Source: CAD feature listing. Evaluate the final solid. Frame: model axes, mm. Coordinates: 2 decimals unless noted, no trailing zeros. Loops run counter-clockwise (first coordinate to the right, second up) from the corner with the lowest first, then second, coordinate; pieces in that order, holes last. Notation, with made-up numbers: (65, -34.5) -> (83, -34.5) arc R19 ccw to (83, -24.5) -> close; hole circle Ø11 at (80.25, -35.75). An arc over 180 degrees is marked (long way). Answer as CSV lines item,"result".
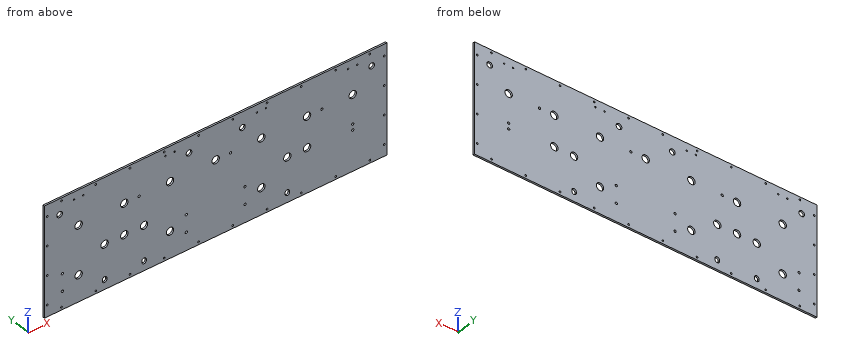
from build123d import *

# Parameters (mm, degrees)
SKETCH1_W           = 600
SKETCH1_H           = 190
EXTRUDE1_DEPTH      = 3
SKETCH2_R           = 6.5
CUT_EXTRUDE1_DEPTH  = 614.929149007
SKETCH5_R           = 2
CUT_EXTRUDE3_DEPTH  = 614.929149007
SKETCH8_R           = 6.5
SKETCH8_R_2         = 2
CUT_EXTRUDE4_DEPTH  = 614.929149007
SKETCH10_R          = 6.5
CUT_EXTRUDE5_DEPTH  = 614.929149007
SKETCH12_R          = 6.5
CUT_EXTRUDE6_DEPTH  = 614.929149007
SKETCH14_R          = 1.25
CUT_EXTRUDE7_DEPTH  = 614.929149007
SKETCH15_R          = 5
CUT_EXTRUDE8_DEPTH  = 614.929149007
CUT_EXTRUDE10_DEPTH = 614.929149007
SKETCH25_R          = 1.5
CUT_EXTRUDE11_DEPTH = 614.929149007
LPATTERN1_COUNT     = 10
LPATTERN1_PITCH     = 60
SKETCH26_R          = 1.5
CUT_EXTRUDE12_DEPTH = 614.929149007
SKETCH27_R          = 2
CUT_EXTRUDE13_DEPTH = 614.929149007


with BuildPart() as part:
    # Sketch1 → Extrude1 (new body)
    with BuildSketch(Plane(origin=(0, 0, 0), x_dir=(1, 0, 0), z_dir=(0, 1, 0))):
        with Locations((300, 35)):
            Rectangle(SKETCH1_W, SKETCH1_H)
    extrude(amount=EXTRUDE1_DEPTH)

    # Sketch2 → Cut-Extrude1 (cut, through all)
    with BuildSketch(Plane(origin=(0, 3, 0), x_dir=(-1, 0, 0), z_dir=(0, 1, 0))):
        with Locations(Location((-60, 0, 0), (0, 0, 90))):
            Circle(SKETCH2_R)
        with Locations(Location((-140, 0, 0), (0, 0, 90))):
            Circle(SKETCH2_R)
        with Locations(Location((-220, 0, 0), (0, 0, 90))):
            Circle(SKETCH2_R)
        with Locations(Location((-300, 0, 0), (0, 0, 90))):
            Circle(SKETCH2_R)
        with Locations(Location((-380, 0, 0), (0, 0, 90))):
            Circle(SKETCH2_R)
        with Locations(Location((-460, 0, 0), (0, 0, 90))):
            Circle(SKETCH2_R)
        with Locations(Location((-540, 0, 0), (0, 0, 90))):
            Circle(SKETCH2_R)
    extrude(amount=-CUT_EXTRUDE1_DEPTH, mode=Mode.SUBTRACT)

    # Sketch5 → Cut-Extrude3 (cut, through all)
    with BuildSketch(Plane(origin=(0, 3, 0), x_dir=(-1, 0, 0), z_dir=(0, 1, 0))):
        with Locations(Location((-166, 0, 0), (0, 0, 90))):
            Circle(SKETCH5_R)
        with Locations(Location((-326, 0, 0), (0, 0, 90))):
            Circle(SKETCH5_R)
        with Locations(Location((-486, 0, 0), (0, 0, 90))):
            Circle(SKETCH5_R)
    extrude(amount=-CUT_EXTRUDE3_DEPTH, mode=Mode.SUBTRACT)

    # Sketch8 → Cut-Extrude4 (cut, through all)
    with BuildSketch(Plane(origin=(0, 3, 0), x_dir=(-1, 0, 0), z_dir=(0, 1, 0))):
        with Locations(Location((-105.461363383, -53.228417592, 0), (0, 0, 90))):
            Circle(SKETCH8_R)
        with Locations(Location((-540, -60, 0), (0, 0, 90))):
            Circle(SKETCH8_R_2)
        with Locations(Location((-425.461363383, -53.228417592, 0), (0, 0, 90))):
            Circle(SKETCH8_R)
        with Locations(Location((-174.538636617, -53.228417592, 0), (0, 0, 90))):
            Circle(SKETCH8_R)
        with Locations(Location((-540, -50, 0), (0, 0, 90))):
            Circle(SKETCH8_R_2)
    extrude(amount=-CUT_EXTRUDE4_DEPTH, mode=Mode.SUBTRACT)

    # Sketch10 → Cut-Extrude5 (cut, through all)
    with BuildSketch(Plane(origin=(0, 3, 0), x_dir=(-1, 0, 0), z_dir=(0, 1, 0))):
        with Locations(Location((-60, -84.184264202, 0), (0, 0, 90))):
            Circle(SKETCH10_R)
        with Locations(Location((-220, -84.184264202, 0), (0, 0, 90))):
            Circle(SKETCH10_R)
        with Locations(Location((-380, -84.184264202, 0), (0, 0, 90))):
            Circle(SKETCH10_R)
    extrude(amount=-CUT_EXTRUDE5_DEPTH, mode=Mode.SUBTRACT)

    # Sketch12 → Cut-Extrude6 (cut, through all)
    with BuildSketch(Plane(origin=(0, 3, 0), x_dir=(-1, 0, 0), z_dir=(0, 1, 0))):
        with Locations(Location((-140, -53.228417592, 0), (0, 0, 90))):
            Circle(SKETCH12_R)
        with Locations(Location((-460, -53.228417592, 0), (0, 0, 90))):
            Circle(SKETCH12_R)
    extrude(amount=-CUT_EXTRUDE6_DEPTH, mode=Mode.SUBTRACT)

    # Sketch14 → Cut-Extrude7 (cut, through all)
    with BuildSketch(Plane(origin=(0, 3, 0), x_dir=(-1, 0, 0), z_dir=(0, 1, 0))):
        with Locations(Location((-52, 47, 0), (0, 0, 90))):
            Circle(SKETCH14_R)
        with Locations(Location((-68, 47, 0), (0, 0, 90))):
            Circle(SKETCH14_R)
        with Locations(Location((-212, 47, 0), (0, 0, 90))):
            Circle(SKETCH14_R)
        with Locations(Location((-228, 47, 0), (0, 0, 90))):
            Circle(SKETCH14_R)
        with Locations(Location((-372, 47, 0), (0, 0, 90))):
            Circle(SKETCH14_R)
        with Locations(Location((-388, 47, 0), (0, 0, 90))):
            Circle(SKETCH14_R)
        with Locations(Location((-532, 47, 0), (0, 0, 90))):
            Circle(SKETCH14_R)
        with Locations(Location((-548, 47, 0), (0, 0, 90))):
            Circle(SKETCH14_R)
    extrude(amount=-CUT_EXTRUDE7_DEPTH, mode=Mode.SUBTRACT)

    # Sketch15 → Cut-Extrude8 (cut, through all)
    with BuildSketch(Plane(origin=(0, 3, 0), x_dir=(-1, 0, 0), z_dir=(0, 1, 0))):
        with Locations(Location((-573.234018716, 33.234018716, 0), (0, 0, 90))):
            Circle(SKETCH15_R)
        with Locations(Location((-26.765981284, 33.234018716, 0), (0, 0, 90))):
            Circle(SKETCH15_R)
        with Locations(Location((-253.234018716, 33.234018716, 0), (0, 0, 90))):
            Circle(SKETCH15_R)
        with Locations(Location((-346.765981284, 33.234018716, 0), (0, 0, 90))):
            Circle(SKETCH15_R)
    extrude(amount=-CUT_EXTRUDE8_DEPTH, mode=Mode.SUBTRACT)

    # Sketch23 → Cut-Extrude10 (cut, through all)
    with BuildSketch(Plane(origin=(0, 3, 0), x_dir=(-1, 0, 0), z_dir=(0, 1, 0))):
        with BuildLine():
            Line((-101.461363383, -112.228417592), (-101.461363383, -114.228417592))
            ThreePointArc((-101.461363383, -114.228417592), (-105.461363383, -118.228417592), (-109.461363383, -114.228417592))
            Line((-109.461363383, -114.228417592), (-109.461363383, -112.228417592))
            ThreePointArc((-109.461363383, -112.228417592), (-105.461363383, -108.228417592), (-101.461363383, -112.228417592))
        make_face()
        with BuildLine():
            Line((-170.538636617, -112.228417592), (-170.538636617, -114.228417592))
            ThreePointArc((-170.538636617, -114.228417592), (-174.538636617, -118.228417592), (-178.538636617, -114.228417592))
            Line((-178.538636617, -114.228417592), (-178.538636617, -112.228417592))
            ThreePointArc((-178.538636617, -112.228417592), (-174.538636617, -108.228417592), (-170.538636617, -112.228417592))
        make_face()
        with BuildLine():
            Line((-421.461363383, -112.228417592), (-421.461363383, -114.228417592))
            ThreePointArc((-421.461363383, -114.228417592), (-425.461363383, -118.228417592), (-429.461363383, -114.228417592))
            Line((-429.461363383, -114.228417592), (-429.461363383, -112.228417592))
            ThreePointArc((-429.461363383, -112.228417592), (-425.461363383, -108.228417592), (-421.461363383, -112.228417592))
        make_face()
    extrude(amount=-CUT_EXTRUDE10_DEPTH, mode=Mode.SUBTRACT)

    # Sketch25 → Cut-Extrude11 (cut, through all)
    with BuildSketch(Plane(origin=(0, 3, 0), x_dir=(-1, 0, 0), z_dir=(0, 1, 0))):
        with Locations(Location((-30, 55, 0), (0, 0, 90))):
            Circle(SKETCH25_R)
        with Locations(Location((-30, -125, 0), (0, 0, 90))):
            Circle(SKETCH25_R)
    cut_extrude11 = extrude(amount=-CUT_EXTRUDE11_DEPTH, mode=Mode.SUBTRACT)

    # LPattern1: Cut-Extrude11 ×10
    with Locations(*[(i * LPATTERN1_PITCH, 0, 0) for i in range(1, LPATTERN1_COUNT)]):
        add(cut_extrude11, mode=Mode.SUBTRACT)

    # Sketch26 → Cut-Extrude12 (cut, through all)
    with BuildSketch(Plane(origin=(0, 3, 0), x_dir=(-1, 0, 0), z_dir=(0, 1, 0))):
        with Locations(Location((-5, -110, 0), (0, 0, 90))):
            Circle(SKETCH26_R)
        with Locations(Location((-5, -60, 0), (0, 0, 90))):
            Circle(SKETCH26_R)
        with Locations(Location((-5, 40, 0), (0, 0, 90))):
            Circle(SKETCH26_R)
        with Locations(Location((-5, -10, 0), (0, 0, 90))):
            Circle(SKETCH26_R)
        with Locations(Location((-595, -110, 0), (0, 0, 90))):
            Circle(SKETCH26_R)
        with Locations(Location((-595, -60, 0), (0, 0, 90))):
            Circle(SKETCH26_R)
        with Locations(Location((-595, -10, 0), (0, 0, 90))):
            Circle(SKETCH26_R)
        with Locations(Location((-595, 40, 0), (0, 0, 90))):
            Circle(SKETCH26_R)
    extrude(amount=-CUT_EXTRUDE12_DEPTH, mode=Mode.SUBTRACT)

    # Sketch27 → Cut-Extrude13 (cut, through all)
    with BuildSketch(Plane(origin=(0, 3, 0), x_dir=(-1, 0, 0), z_dir=(0, 1, 0))):
        with Locations(Location((-351.5, -99.041033847, 0), (0, 0, 90))):
            Circle(SKETCH27_R)
        with Locations(Location((-351.5, -69.041033847, 0), (0, 0, 90))):
            Circle(SKETCH27_R)
        with Locations(Location((-248.5, -99.041033847, 0), (0, 0, 90))):
            Circle(SKETCH27_R)
        with Locations(Location((-248.5, -69.041033847, 0), (0, 0, 90))):
            Circle(SKETCH27_R)
        with Locations(Location((-31.498394821, -99.041033847, 0), (0, 0, 90))):
            Circle(SKETCH27_R)
        with Locations(Location((-31.498394821, -69.041033847, 0), (0, 0, 90))):
            Circle(SKETCH27_R)
    extrude(amount=-CUT_EXTRUDE13_DEPTH, mode=Mode.SUBTRACT)


solid = part.part
(1) Material intervals for L1, parallel to Z at x = 210, y = 0.6; L2, parallel to X at y = 1.3, z = -10; L3, parallel to Z at x = 486, y = 0.8, sorted ascending. Write a range as [from, to].
Computed values:
L1,"[-130, -126.5], [-123.5, 53.5], [56.5, 60]"
L2,"[0, 3.5], [6.5, 593.5], [596.5, 600]"
L3,"[-130, -2], [2, 60]"
(2) Cut plane B-B (y = 0.95). State how many separate pieces and enclosed holes the cut face has, then the cut area to 3 significant figures.
Computed values:
separate pieces,"1"
enclosed holes,"69"
area,"111,000 mm^2"
(3) Pin query (flat end, axial travel): pin 1 Ø3.5 at (x, z) = (31.5, -99.04) entering from -Y. Return the tip coordinate at first contact, or that it passes through.
Computed values:
pin 1,"through"
(4) Cut plane A-A (x = 380). Return the cut outline in (y, z), then the cut area to 3 significant figures.
Computed values:
outline,"(0, -130) -> (3, -130) -> (3, -90.68) -> (0, -90.68) -> close; (0, -77.68) -> (3, -77.68) -> (3, -6.5) -> (0, -6.5) -> close; (0, 6.5) -> (3, 6.5) -> (3, 60) -> (0, 60) -> close"
area,"492 mm^2"
